from build123d import *

# Parameters (mm, degrees)
SKETCH1_R                = 6.5
BOSS_EXTRUDE1_DEPTH      = 53.4
SKETCH11_R               = 4.875
BOSS_EXTRUDE2_DEPTH      = 20
BOSS_EXTRUDE3_START      = 20
SKETCH12_R               = 4.875
BOSS_EXTRUDE3_DEPTH      = 20
CIRPATTERN1_COUNT        = 2
BOSS_EXTRUDE4_DEPTH      = 26.7
BOSS_EXTRUDE4_DEPTH_BACK = 26.7
SKETCH13_R               = 6.5
SKETCH14_R               = 4.875
BOSS_EXTRUDE5_DEPTH      = 10
BOSS_EXTRUDE6_START      = 10
SKETCH15_R               = 4.875
BOSS_EXTRUDE6_DEPTH      = 10


with BuildPart() as part:
    # Sketch1 → Boss-Extrude1 (new body)
    with BuildSketch(Plane(origin=(0, 0, 0), x_dir=(1, 0, 0), z_dir=(0, 1, 0))):
        with Locations(Location((0, 0, 0), (0, 0, 270))):
            Circle(SKETCH1_R)
    boss_extrude1 = extrude(amount=BOSS_EXTRUDE1_DEPTH)

    # Sketch11 → Boss-Extrude2 (add)
    with BuildSketch(Plane(origin=(0, 0, 0), x_dir=(-1, 0, 0), z_dir=(0, -1, 0))):
        with Locations(Location((0, 0, 0), (0, 0, 90))):
            Circle(SKETCH11_R)
    boss_extrude2 = extrude(amount=BOSS_EXTRUDE2_DEPTH)

    # Sketch12 → Boss-Extrude3 (add)
    with BuildSketch(Plane(origin=(0, 53.4, 0), x_dir=(1, 0, 0), z_dir=(0, 1, 0)).offset(BOSS_EXTRUDE3_START)):
        with Locations(Location((0, 0, 0), (0, 0, 90))):
            Circle(SKETCH12_R)
    boss_extrude3 = extrude(amount=-BOSS_EXTRUDE3_DEPTH)


with BuildPart() as cirpattern1_1:
    # CirPattern1: Boss-Extrude1, Boss-Extrude2, Boss-Extrude3 ×2 about axis
    cirpattern1_axis = Axis((0, 26.7, 0), (1, 0, 0))
    add([boss_extrude1.rotate(cirpattern1_axis, i * 360 / CIRPATTERN1_COUNT) for i in range(1, CIRPATTERN1_COUNT)])
    add([boss_extrude2.rotate(cirpattern1_axis, i * 360 / CIRPATTERN1_COUNT) for i in range(1, CIRPATTERN1_COUNT)])
    add([boss_extrude3.rotate(cirpattern1_axis, i * 360 / CIRPATTERN1_COUNT) for i in range(1, CIRPATTERN1_COUNT)])


with BuildPart() as part_1:
    add(part.part)

    # CirPattern1 united with what the copies: union CirPattern1_1
    add(cirpattern1_1.part)

    # Sketch13 → Boss-Extrude4 (add, two sides: drawn at the far end of the back side and taken through both)
    with BuildSketch(Plane(origin=(0, 0, 0), x_dir=(-1, 0, 0), z_dir=(0, 0, -1)).offset(-BOSS_EXTRUDE4_DEPTH_BACK)):
        with Locations((0, 26.7)):
            Circle(SKETCH13_R)
    extrude(amount=BOSS_EXTRUDE4_DEPTH + BOSS_EXTRUDE4_DEPTH_BACK)

    # Sketch14 → Boss-Extrude5 (add)
    with BuildSketch(Plane(origin=(0, 0, -26.7), x_dir=(-1, 0, 0), z_dir=(0, 0, -1))):
        with Locations((0, 26.7)):
            Circle(SKETCH14_R)
    extrude(amount=BOSS_EXTRUDE5_DEPTH)

    # Sketch15 → Boss-Extrude6 (add)
    with BuildSketch(Plane.XY.offset(26.7).offset(BOSS_EXTRUDE6_START)):
        with Locations(Location((0, 26.7, 0), (0, 0, 180))):
            Circle(SKETCH15_R)
    extrude(amount=-BOSS_EXTRUDE6_DEPTH)


solid = part_1.part
Read the model definition and answer for the solid it produces. Units are mm, in the model's axes. A direction names the side the tool comes from. Coordinates: 2 decimals unless noted, no trailing zeros. Write each loop counter-clockwise with the first axis right and the second up, starting at its lowest first coordinate (ties: lowest second). Pieces come first, ordered by that corner, then holes. Notation, with made-up numbers: (-30, -16) - (2, -16) arc R20 ccw to (2, -6) - close; hole circle Ø8 at (55, 85). An arc over 180 degrees is marked (long way). One line per question, with ' | ' between items.
Q1. For faces 1 (the cylindrical face through (1.06, 21.94, -31.63)), 2 (the flat face through (5, 53.4, 1)), 3 (the cylindrical face through (6.494, 26.986, 16.504)), 4 (the flat face through (0, 27, 36.7)), 5 (the cylindrical face through (4.834, -9.86, 0.635)), determine the directions among +Z, -Z, +X, -X, +Y, -Y from which every point of the face is accessible in a straight line to the end or side of a thin tool.
Result set:
face 1: -Z | face 2: +Y | face 3: +Z | face 4: +Z, +X, -X, +Y, -Y | face 5: -Y
Q2. Find section A-A, the plane x = 0. Write down the section's boundary in (y, z) (3 decimals), plus the area to 3 significant figures.
Result set:
outline: (-20, -4.875) - (0, -4.875) - (0, -6.5) - (20.2, -6.5) - (20.2, -26.7) - (21.825, -26.7) - (21.825, -36.7) - (31.575, -36.7) - (31.575, -26.7) - (33.2, -26.7) - (33.2, -6.5) - (53.4, -6.5) - (53.4, -4.875) - (73.4, -4.875) - (73.4, 4.875) - (53.4, 4.875) - (53.4, 6.5) - (33.2, 6.5) - (33.2, 26.7) - (31.575, 26.7) - (31.575, 36.7) - (21.825, 36.7) - (21.825, 26.7) - (20.2, 26.7) - (20.2, 6.5) - (0, 6.5) - (0, 4.875) - (-20, 4.875) - close | area: 1,800 mm^2
Q3. Consider L1, parallel to Y at x = -0.5, z = -12.5; L2, parallel to Y at x = -1.75, z = 6; L3, parallel to X at y = 23, z = -31.5. Determine where each line is inside the solid, lowest interval first. Write a range as [from, to].
Result set:
L1: [20.22, 33.18] | L2: [0, 53.4] | L3: [-3.17, 3.17]
Q4. Each of these flat-tipped pins is pushed along its axis until it touches: P1, Ø3, axis at x = -0.5, z = -27, coming from the +Y side; P2, Ø12, axis at y = 42.5, z = -10.5, coming from the -X side; P3, Ø12, axis at y = 33.5, z = 15.5, coming from the +X side. Where does it stop, or does it pass through?
Result set:
P1: y = 33.2 | P2: x = -4.69 | P3: x = 6.45
Q5. Find section B-B, the plane z = 11. Write down the section's boundary in (x, y), plus the area to 3 significant figures.
Result set:
outline: circle Ø13 at (0, 26.7) | area: 133 mm^2
Q6. Find section C-C, the plane y = 62. Write down the section's boundary in (x, z) (3 decimals), plus the area to 3 significant figures.
Result set:
outline: circle Ø9.75 at (0, 0) | area: 74.7 mm^2
